Geometry: final body of the model. Coordinates: model frame, mm. A direction names the side the tool comes from. Give positions to 0.01 mm unless a question says otherwise; leave off trailing zeros. Loops run counter-clockwise (first coordinate to the right, second up) from the corner with the lowest first, then second, coordinate; pieces in that order, holes last.
from build123d import *

# Parameters (mm, degrees)
CROQUIS1_R              = 34
CROQUIS1_R_2            = 1.5
SALIENTE_EXTRUIR1_DEPTH = 4
CORTAR_EXTRUIR1_DEPTH   = 4
SALIENTE_EXTRUIR2_START = 6
CROQUIS3_R              = 9
CROQUIS3_R_2            = 1.5
SALIENTE_EXTRUIR2_DEPTH = 6


with BuildPart() as part:
    # Croquis1 → Saliente-Extruir1 (new body)
    with BuildSketch(Plane.XY):
        Circle(CROQUIS1_R)
        with Locations((0, 25)):
            Circle(CROQUIS1_R_2, mode=Mode.SUBTRACT)
        with Locations((21.650635095, -12.5)):
            Circle(CROQUIS1_R_2, mode=Mode.SUBTRACT)
        with Locations((-21.650635095, -12.5)):
            Circle(CROQUIS1_R_2, mode=Mode.SUBTRACT)
    extrude(amount=SALIENTE_EXTRUIR1_DEPTH)

    # Croquis2 → Cortar-Extruir1 (cut)
    with BuildSketch(Plane(origin=(0, 0, 0), x_dir=(-1, 0, 0), z_dir=(0, 0, -1))):
        Polygon((3.550704156, 6.15), (-3.550704156, 6.15), (-7.101408311, 0), (-3.550704156, -6.15), (3.550704156, -6.15), (7.101408311, 0), align=None)
    extrude(amount=-CORTAR_EXTRUIR1_DEPTH, mode=Mode.SUBTRACT)

    # Croquis3 → Saliente-Extruir2 (add)
    # profile 1 of 4: a face of its own
    with BuildSketch(Plane(origin=(0, 0, 0), x_dir=(-1, 0, 0), z_dir=(0, 0, -1)).offset(SALIENTE_EXTRUIR2_START)):
        with Locations(Location((0, 0, 0), (0, 0, 180))):
            Circle(CROQUIS3_R)
        Polygon((-7.101408311, 0), (-3.550704156, 6.15), (3.550704156, 6.15), (7.101408311, 0), (3.550704156, -6.15), (-3.550704156, -6.15), align=None, mode=Mode.SUBTRACT)
    # profile 2 of 4: a face of its own
    with BuildSketch(Plane(origin=(0, 0, 0), x_dir=(-1, 0, 0), z_dir=(0, 0, -1)).offset(SALIENTE_EXTRUIR2_START)):
        with Locations(Location((0, 25, 0), (0, 0, 180))):
            Circle(CROQUIS3_R_2)
    # profile 3 of 4: a face of its own
    with BuildSketch(Plane(origin=(0, 0, 0), x_dir=(-1, 0, 0), z_dir=(0, 0, -1)).offset(SALIENTE_EXTRUIR2_START)):
        with Locations(Location((-21.650635095, -12.5, 0), (0, 0, 180))):
            Circle(CROQUIS3_R_2)
    # profile 4 of 4: a face of its own
    with BuildSketch(Plane(origin=(0, 0, 0), x_dir=(-1, 0, 0), z_dir=(0, 0, -1)).offset(SALIENTE_EXTRUIR2_START)):
        with Locations(Location((21.650635095, -12.5, 0), (0, 0, 180))):
            Circle(CROQUIS3_R_2)
    extrude(amount=-SALIENTE_EXTRUIR2_DEPTH)


with BuildPart() as saliente_extruir2_kept_piece:
    # of the separate pieces the step leaves, the one the design keeps (saliente_extruir2_pieces_kept)
    add(part.part.solids().sort_by_distance((34, 0, 0))[0])

    # Croquis4 → Revolución1 (revolve)
    with BuildSketch(Plane(origin=(0, 0, 0), x_dir=(1, 0, 0), z_dir=(0, 1, 0))):
        Polygon((9, 6), (9, 0), (16.96226893, 0), align=None)
    revolve(axis=Axis((0, 0, -12.759887465), (0, 0, 1)))


solid = saliente_extruir2_kept_piece.part
Item 1: Set-up query: faces 5 (the face through (0, -6.15, -1)), 6 (the face through (4, 6, -6)). Return all of +Z, -Z, +X, -X, +Y, -Y with unobstructed straight access to the full face (end or side cutting, diameter ignored); none if empty.
Values follow:
face 5: +Z, -Z
face 6: -Z, +X, -X, +Y, -Y
Item 2: Pin query (flat end, axial travel): pin 1 (3.5 mm diameter, centred on x = -1.5, z = -1, fed in from -Y); pin 2 (1 mm diameter, centred on y = -13.5, z = 2.5, fed in from -X); pin 3 (2 mm diameter, centred on x = 8.5, y = -21, fed in from -Z); pin 4 (2.5 mm diameter, centred on x = -21.65, y = -12.5, fed in from +Z). Return the tip coordinate at first contact, or that it passes through.
Values follow:
pin 1: stops at y = -34
pin 2: stops at x = -31.42
pin 3: stops at z = 0
pin 4: passes through
Item 3: Draft query along X for faces 1 (the face through (18.28, 28.67, 1.97)), 2 (the face through (-20.22, -12.05, 1.97)), 3 (the face through (-16, -7, 0)), 4 (the face through (0, 6.15, -1)). Return one class per face: +X half, -X half, draft (parallel to the pull), parting line (faces both ways), or undercut.
Values follow:
face 1: parting line
face 2: undercut
face 3: draft
face 4: undercut
Item 4: Section query D-D on y = -12.5. Give the number of separate pieces and of enclosed holes in the cut face, plus the area to 3 significant figures.
Values follow:
separate pieces: 3
enclosed holes: 0
area: 279 mm2
Item 5: Section query C-C on z = -2.5. Return loops of the section in (x, y), plus the area to 3 significant figures.
Values follow:
outline: circle Ø27.29 at (0, 0); hole (-7.1, 0) - (-3.55, -6.15) - (3.55, -6.15) - (7.1, 0) - (3.55, 6.15) - (-3.55, 6.15) - close
area: 454 mm2
Item 6: Ray query, probe 1 along Y at (x, z) = (0, 0.95); probe 2 along Z at (x, y) = (-20, 10.5); probe 3 along X at (y, z) = (-1.5, -3). Return the intervals inside material, ascending.
Values follow:
probe 1: y = -34 to -6.15, 6.15 to 23.5, 26.5 to 34
probe 2: z = 0 to 4
probe 3: x = -12.89 to -6.24, 6.24 to 12.89
Item 7: Section query A-A on x = 0. Return loops of the section in (y, z), plus the area to 3 significant figures.
Values follow:
outline: (-34, 0) - (-16.96, 0) - (-9, -6) - (-6.15, -6) - (-6.15, 4) - (-34, 4) - close; (6.15, -6) - (9, -6) - (16.96, 0) - (23.5, 0) - (23.5, 4) - (6.15, 4) - close; (26.5, 0) - (34, 0) - (34, 4) - (26.5, 4) - close
area: 293 mm2
Item 8: Section query B-B on z = 1.5. Return loops of the section in (x, y), plus the area to 3 significant figures.
Values follow:
outline: circle Ø68 at (0, 0); hole circle Ø3 at (-21.65, -12.5); hole (-7.1, 0) - (-3.55, -6.15) - (3.55, -6.15) - (7.1, 0) - (3.55, 6.15) - (-3.55, 6.15) - close; hole circle Ø3 at (0, 25); hole circle Ø3 at (21.65, -12.5)
area: 3,480 mm2
